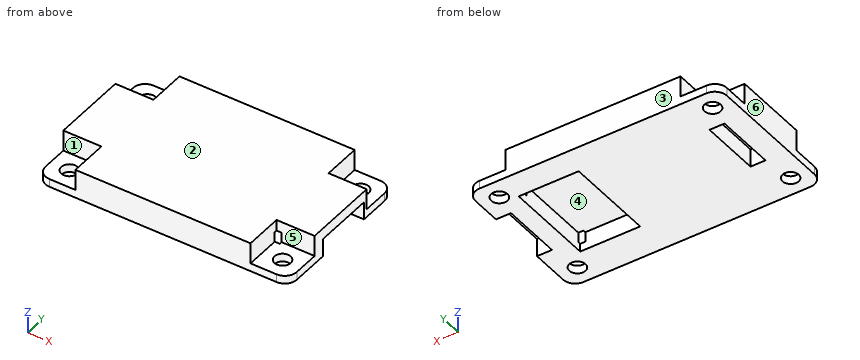
```python
from build123d import *

# Parameters (mm, degrees)
SKETCH1_R           = 1.35
BOSS_EXTRUDE1_DEPTH = 4.85
SKETCH2_W           = 2.5
SKETCH2_H           = 10
SKETCH2_W_2         = 10
SKETCH2_H_2         = 15
CUT_EXTRUDE1_DEPTH  = 3
SKETCH4_W           = 6.35
SKETCH4_H           = 6.35
CUT_EXTRUDE3_DEPTH  = 3.5


with BuildPart() as part:
    # Sketch1 → Boss-Extrude1 (new body)
    with BuildSketch(Plane.XY):
        with BuildLine():
            Line((-2, 0), (-39.91, 0))
            ThreePointArc((-39.91, 0), (-41.324213562, -0.585786438), (-41.91, -2))
            Line((-41.91, -2), (-41.91, -23.4))
            ThreePointArc((-41.91, -23.4), (-41.324213562, -24.814213562), (-39.91, -25.4))
            Line((-39.91, -25.4), (-2, -25.4))
            ThreePointArc((-2, -25.4), (-0.585786438, -24.814213562), (0, -23.4))
            Line((0, -23.4), (0, -2))
            ThreePointArc((0, -2), (-0.585786438, -0.585786438), (-2, 0))
        make_face()
        with Locations(Location((-38.735, -22.225, 0), (0, 0, 180))):
            Circle(SKETCH1_R, mode=Mode.SUBTRACT)
        with Locations(Location((-38.735, -3.175, 0), (0, 0, 180))):
            Circle(SKETCH1_R, mode=Mode.SUBTRACT)
        with Locations(Location((-3.175, -3.175, 0), (0, 0, 180))):
            Circle(SKETCH1_R, mode=Mode.SUBTRACT)
        with Locations(Location((-3.175, -22.225, 0), (0, 0, 180))):
            Circle(SKETCH1_R, mode=Mode.SUBTRACT)
    extrude(amount=BOSS_EXTRUDE1_DEPTH)

    # Sketch2 → Cut-Extrude1 (cut)
    with BuildSketch(Plane(origin=(0, 0, 0), x_dir=(-1, 0, 0), z_dir=(0, 0, -1))):
        with Locations((1.25, -12)):
            Rectangle(SKETCH2_W, SKETCH2_H)
        with Locations((10.5, -12)):
            Rectangle(SKETCH2_W_2, SKETCH2_H_2)
        with Locations((36.86, -12)):
            Rectangle(SKETCH2_W, SKETCH2_H)
    extrude(amount=-CUT_EXTRUDE1_DEPTH, mode=Mode.SUBTRACT)

    # Sketch4 → Cut-Extrude3 (cut)
    with BuildSketch(Plane.XY.offset(4.85)):
        with Locations((-38.735, -3.175)):
            Rectangle(SKETCH4_W, SKETCH4_H)
        with Locations((-38.735, -22.225)):
            Rectangle(SKETCH4_W, SKETCH4_H)
        with Locations((-3.175, -22.225)):
            Rectangle(SKETCH4_W, SKETCH4_H)
        with Locations((-3.175, -3.175)):
            Rectangle(SKETCH4_W, SKETCH4_H)
    extrude(amount=-CUT_EXTRUDE3_DEPTH, mode=Mode.SUBTRACT)


solid = part.part
```
Design review of the part built by this model. Coordinates are the model's own, in mm. Face numbers are marked on the shaded views. A direction names the side the tool comes from. Coordinates: 2 decimals unless noted, no trailing zeros. Order: outer loops, then holes, each group sorted by start corner. A loop starts at its lowest first (then second) coordinate and runs counter-clockwise, first axis right, second up. Notation, with made-up numbers: (-0.75, 51.25) - (55.25, 51.25) arc R3 cw to (55.25, 56.25) - close; hole circle Ø10 at (89.5, 24.5). An arc over 180 degrees is marked (long way). Answer in a Markdown table with one row per item.
(1) Wall thickness on line 1 along X through (y, z) = (-22.25, 0.65); line 2 along X through (y, z) = (-7.75, 1.25); line 3 along Y through (x, z) = (-37, 3.55): over which ranges is each line inside the solid? List them lowest first. Write a range as from..to.
Checked values:
| item | result |
|---|---|
| line 1 | -41.91..-40.08, -37.39..-4.52, -1.83..0 |
| line 2 | -41.91..-38.11, -35.61..-15.5, -5.5..-2.5 |
| line 3 | -19.05..-6.35 |
(2) The part is to be moulded in two halves that separate along Y. For the marked faces 3, 4, 5 and 6, say which applies: released by +Y, released by -Y, zero draft, split by the parting line, or undercut.
Checked values:
| item | result |
|---|---|
| face 3 | released by +Y |
| face 4 | undercut |
| face 5 | released by -Y |
| face 6 | zero draft |
(3) Consider section A-A on z = 2.3. State the section outline as (x, y) points.
Checked values:
| item | result |
|---|---|
| outline | (-41.91, -19.05) - (-35.56, -19.05) - (-35.56, -25.4) - (-6.35, -25.4) - (-6.35, -19.5) - (-15.5, -19.5) - (-15.5, -4.5) - (-6.35, -4.5) - (-6.35, 0) - (-35.56, 0) - (-35.56, -6.35) - (-41.91, -6.35) - close; (-5.5, -19.05) - (0, -19.05) - (0, -17) - (-2.5, -17) - (-2.5, -7) - (0, -7) - (0, -6.35) - (-5.5, -6.35) - close; hole (-38.11, -17) - (-35.61, -17) - (-35.61, -7) - (-38.11, -7) - close |
(4) For the marked faces 1 and 2, list the 3-axis set-ups (+Z, -Z, +X, -X, +Y, -Y) from which the entire face can be reached by the end or side of a thin tool; tool diameter is ignored.
Checked values:
| item | result |
|---|---|
| face 1 | +Z, -X, -Y |
| face 2 | +Z, +X, -X, +Y, -Y |
(5) Clearance check with flat-ended pins moving along their axes: pin 1 (1 mm diameter, centred on y = -2.5, z = 4, fed in from +X); pin 2 (0.9 mm diameter, centred on y = -10.5, z = 1, fed in from +X); pin 3 (3 mm diameter, centred on x = -40, y = -22, fed in from +Z); pin 4 (2.5 mm diameter, centred on x = -38.735, y = -22.225, fed in from -Z). State where each tip first meets the part, or that it passes through.
Checked values:
| item | result |
|---|---|
| pin 1 | x = -6.35 |
| pin 2 | x = -2.5 |
| pin 3 | z = 1.35 |
| pin 4 | through |
(6) Consider section B-B on y = -16.5. State the section outline as (x, z) points, plus the area to 3 significant figures.
Checked values:
| item | result |
|---|---|
| outline | (-41.91, 0) - (-38.11, 0) - (-38.11, 3) - (-35.61, 3) - (-35.61, 0) - (-15.5, 0) - (-15.5, 3) - (-5.5, 3) - (-5.5, 0) - (-2.5, 0) - (-2.5, 3) - (0, 3) - (0, 4.85) - (-41.91, 4.85) - close |
| area | 158 mm^2 |
(7) Consider section D-D on y = -21.5. State the section outline as (x, z) points, plus the area to 3 significant figures.
Checked values:
| item | result |
|---|---|
| outline | (-41.91, 0) - (-39.87, 0) - (-39.87, 1.35) - (-41.91, 1.35) - close; (-37.6, 0) - (-4.31, 0) - (-4.31, 1.35) - (-6.35, 1.35) - (-6.35, 4.85) - (-35.56, 4.85) - (-35.56, 1.35) - (-37.6, 1.35) - close; (-2.04, 0) - (0, 0) - (0, 1.35) - (-2.04, 1.35) - close |
| area | 153 mm^2 |
(8) Consider section C-C on x = -4. State the section outline as (y, z) points.
Checked values:
| item | result |
|---|---|
| outline | (-25.4, 0) - (-23.29, 0) - (-23.29, 1.35) - (-25.4, 1.35) - close; (-21.16, 0) - (-4.24, 0) - (-4.24, 1.35) - (-6.35, 1.35) - (-6.35, 4.85) - (-19.05, 4.85) - (-19.05, 1.35) - (-21.16, 1.35) - close; (-2.11, 0) - (0, 0) - (0, 1.35) - (-2.11, 1.35) - close |
